For this review, take the finished solid that the model builds, in its own axes (mm). A direction names the side the tool comes from. Give positions to 0.01 mm unless a question says otherwise; leave off trailing zeros. Write each loop counter-clockwise with the first axis right and the second up, starting at its lowest first coordinate (ties: lowest second). Pieces come first, ordered by that corner, then holes.
Q1. Mouldability with a two-part tool opening along X and no side actions: class faces 4 (the conical face through (842.046, 6028.379, 11.443)), 5 (the flat face through (832, 5940.625, 5)), 6 (the flat face through (838.696, 5949.759, 11.61)) as released by +X, released by -X, zero draft, split by the parting line, or undercut.
Q2. We need section C-C (y = 6126.5). Write out the cut boundary in (x, z) (1 decimal), then the cut area to 3 significant figures.
Q3. We need section B-B (x = 865). Write out the cut boundary in (y, z) (3 decimals), then the cut area to 3 significant figures.
Q4. We need section A-A (y = 6048). Write out the cut boundary in (x, z), then the cut area to 3 significant figures.
Q5. For line 1 (Y direction, x = 835.5, z = 5); line 2 (Z direction, x = 841, y = 6138); line 3 (Y direction, x = 852, z = 4), list the stretches that pass through material, from the lowest coordinate up.
Q6. Machinability: for faces 1 (the cylindrical face through (839.37, 6142.44, 6.62)), 2 (the flat face through (864, 6173, 3.175)), 3 (the cylindrical face through (840.82, 6030.12, 4.79)), which of the approach directions +Z, -Z, +X, -X, +Y, -Y give a long, thin tool a straight path to every point of the face, cutting with its end or side? Answer none if there is none.
Q7. Insertion check: P1, Ø1, axis at y = 6009.5, z = 12, coming from the +X side; P2, Ø7, axis at x = 866, y = 6171.5, coming from the +Z side (3 decimals); P3, Ø4.5, axis at x = 830, z = 4.5, coming from the +Y side; P4, Ø5, axis at y = 6017, z = 11, coming from the -X side. Each pin has a flat end and moves straight along its axis. Give the tip position at first contact, or say it passes through.
```python
from build123d import *

# Parameters (mm, degrees)
SKETCH2_W                  = 82.738044028
SKETCH2_H                  = 243.598411898
BOSS_EXTRUDE1_DEPTH        = 3.175
BOSS_EXTRUDE2_DEPTH        = 243.598412
CUT_EXTRUDE1_DEPTH         = 6253.234293578
CUT_EXTRUDE1_DEPTH_BACK    = 6253.234293578
SKETCH3_W                  = 10.058364279
SKETCH3_H                  = 111.125
FILLET1_R                  = 6.35
CUT_EXTRUDE2_DEPTH         = 6243.564603497
DELETEFACE2_START          = 830.447299741
DELETEFACE2_OUTLINE_W      = 243.598411898
DELETEFACE2_OUTLINE_H      = 6
DELETEFACE2_DEPTH          = 0.551332964
F_6_0_204_DIAMETER_HOLE1_D = 5.1816
CUT_EXTRUDE3_START         = 3.175
CUT_EXTRUDE3_DEPTH         = 6231.095925463
SKETCH10_W                 = 38.1
SKETCH10_H                 = 3.175
BOSS_EXTRUDE4_DEPTH        = 6.35
BOSS_EXTRUDE6_DEPTH        = 1.5875
CUT_EXTRUDE4_DEPTH         = 913.829845298
FILLET2_R                  = 9.525
FILLET3_R                  = 3.175
SKETCH13_W                 = 8.255
SKETCH13_H                 = 6.35
BOSS_EXTRUDE5_DEPTH        = 1.5875
FILLET4_R                  = 2.54
FILLET5_SIZE               = 6.35
FILLET5_SIZE_2             = 3.175
FILLET6_R                  = 3.175
HOLE1_AT_2_COUNT           = 2
HOLE1_AT_2_PITCH           = 123.825
HOLE1_AT_3_COUNT           = 2
HOLE1_AT_3_PITCH           = 212.6865263
F_4_CLEARANCE_HOLE1_D      = 3.4544


# Read off the part's stored shape, not the designer's step: DeleteFace2
with BuildPart() as part:
    # Sketch2 → Boss-Extrude1 (new body)
    with BuildSketch(Plane.XY):
        with Locations((870.137648104, 6053.851709568)):
            Rectangle(SKETCH2_W, SKETCH2_H)
    extrude(amount=BOSS_EXTRUDE1_DEPTH)

    # Sketch5 → Boss-Extrude2 (add, through all)
    with BuildSketch(Plane(origin=(0, 6175.650915517, 0), x_dir=(1, 0, 0), z_dir=(0, 1, 0))):
        Polygon((828.76862609, -3.175), (840.781978058, -13.382293294), (845.472124982, -12.555293847), (843.81812609, -3.175), align=None)
    extrude(amount=-BOSS_EXTRUDE2_DEPTH)

    # Sketch3 → Cut-Extrude1 (cut, two sides: drawn at the far end of the back side and taken through both)
    with BuildSketch(Plane(origin=(1789.89403363, 0, -153.971769821), x_dir=(-0.9848077530122082, 0, 0.17364817766692958), z_dir=(-0.17364817766692958, 0, -0.9848077530122082)).offset(-CUT_EXTRUDE1_DEPTH_BACK)):
        with Locations((968.782821029, 6016.190003619)):
            Rectangle(SKETCH3_W, SKETCH3_H)
    extrude(amount=CUT_EXTRUDE1_DEPTH + CUT_EXTRUDE1_DEPTH_BACK, mode=Mode.SUBTRACT)

    # Fillet1
    fillet1_edges = [part.edges().sort_by_distance(p)[0] for p in [
        (839.602148372, 6071.752503619, 6.691146647),
        (839.602148372, 5960.627503619, 6.691146647),
    ]]
    fillet(fillet1_edges, radius=FILLET1_R)

    # Sketch4 → Cut-Extrude2 (cut, through all)
    with BuildSketch(Plane.XY.offset(3.175)):
        Polygon((843.81812609, 6170.570915517), (843.81812609, 6175.650915517), (911.506670118, 6175.650915517), (911.506670118, 5932.052503619), (905.156670118, 5932.052503619), (843.81812609, 5932.052503619), align=None)
    extrude(amount=-CUT_EXTRUDE2_DEPTH, mode=Mode.SUBTRACT)

    # DeleteFace2 outline → DeleteFace2 (cut)
    with BuildSketch(Plane(origin=(0, 0, 0), x_dir=(0, 1, 0), z_dir=(0.984807753012209, 0, -0.173648177666925)).offset(DELETEFACE2_START)):
        with Locations((6053.851709568, 148)):
            Rectangle(DELETEFACE2_OUTLINE_W, DELETEFACE2_OUTLINE_H)
    extrude(amount=DELETEFACE2_DEPTH, mode=Mode.SUBTRACT)

    # #6 (0.204) Diameter Hole1 (through all)
    with Locations(Plane(origin=(0, 0, 0), x_dir=(-1, 0, 0), z_dir=(0, 0, -1))):
        with Locations((-833.65812609, 6161.363415517), (-833.65812609, 6142.313415517), (-833.65812609, 5946.340003619)):
            Hole(F_6_0_204_DIAMETER_HOLE1_D / 2)

    # Sketch8 → Cut-Extrude3 (cut, through all)
    with BuildSketch(Plane.XY.offset(CUT_EXTRUDE3_START)):
        with BuildLine():
            Line((833.65812609, 6155.648415517), (828.76862609, 6155.648415517))
            ThreePointArc((828.76862609, 6155.648415517), (823.05362609, 6161.363415517), (828.76862609, 6167.078415517))
            Line((828.76862609, 6167.078415517), (833.65812609, 6167.078415517))
            ThreePointArc((833.65812609, 6167.078415517), (839.37312609, 6161.363415517), (833.65812609, 6155.648415517))
        make_face()
        with BuildLine():
            Line((833.65812609, 6136.598415517), (828.76862609, 6136.598415517))
            ThreePointArc((828.76862609, 6136.598415517), (823.05362609, 6142.313415517), (828.76862609, 6148.028415517))
            Line((828.76862609, 6148.028415517), (833.65812609, 6148.028415517))
            ThreePointArc((833.65812609, 6148.028415517), (839.37312609, 6142.313415517), (833.65812609, 6136.598415517))
        make_face()
        with BuildLine():
            Line((833.65812609, 5940.625003619), (828.76862609, 5940.625003619))
            ThreePointArc((828.76862609, 5940.625003619), (823.05362609, 5946.340003619), (828.76862609, 5952.055003619))
            Line((828.76862609, 5952.055003619), (833.65812609, 5952.055003619))
            ThreePointArc((833.65812609, 5952.055003619), (839.37312609, 5946.340003619), (833.65812609, 5940.625003619))
        make_face()
    extrude(amount=CUT_EXTRUDE3_DEPTH, mode=Mode.SUBTRACT)

    # Sketch10 → Boss-Extrude4 (add)
    with BuildSketch(Plane(origin=(0, 6175.650915517, 0), x_dir=(1, 0, 0), z_dir=(0, 1, 0))):
        with Locations((862.308287926, -1.5875)):
            Rectangle(SKETCH10_W, SKETCH10_H)
    extrude(amount=-BOSS_EXTRUDE4_DEPTH)

    # Sketch14 → Boss-Extrude6 (add)
    with BuildSketch(Plane(origin=(817.830939253, 0, -144.205660248), x_dir=(-0.17364817766692534, 0, -0.9848077530122089), z_dir=(0.9848077530122089, 0, -0.17364817766692534))):
        Polygon((-149.654244494, 6169.300915517), (-149.654244494, 6175.650915517), (-159.179244494, 6175.650915517), (-159.179244494, 5932.052503619), (-146.430265001, 5932.052503619), (-146.430265001, 6169.300915517), align=None)
    extrude(amount=BOSS_EXTRUDE6_DEPTH)

    # Sketch15 → Cut-Extrude4 (cut, through all)
    with BuildSketch(Plane(origin=(0, 6169.300915517, 0), x_dir=(1, 0, 0), z_dir=(0, 1, 0))):
        Polygon((843.258287926, 0), (844.870277672, 0), (844.821670234, 0.275666482), align=None)
    extrude(amount=-CUT_EXTRUDE4_DEPTH, mode=Mode.SUBTRACT)

    # Fillet2
    # the kernel refuses this fillet: 9.525 mm, written as the material it adds along each edge
    with BuildSketch(Plane(origin=(845.430115836, 6175.650915517, 3.175), x_dir=(1, 0, 0), z_dir=(0, -1, 0))) as fillet2_piece_1:
        with BuildLine():
            CenterArc((11.121110651, 9.525), FILLET2_R, 182.529491184, 87.470508816)
            Line((1.605391454, 9.104627365), (1.41507707, 9.096219913))
            ThreePointArc((1.41507707, 9.096219913), (0.61508985, 4.585393661), (-0.187605877, 0.033079978))
            Line((-0.187605877, 0.033079978), (0, -0.1905))
            Line((0, -0.1905), (11.121110651, -0.1905))
            Line((11.121110651, -0.1905), (11.121110651, 0))
        make_face()
    extrude(amount=6.35)

    # Fillet3
    # the kernel refuses this fillet: 3.175 mm, written as the material it adds along each edge
    with BuildSketch(Plane(origin=(847.03550729, 6169.300915517, 12.279627365), x_dir=(0.9848077530122001, 0, -0.17364817766697505), z_dir=(-0.17364817766697507, 0, -0.9848077530122002))) as fillet3_piece_1_section:
        with BuildLine():
            CenterArc((FILLET3_R, FILLET3_R), FILLET3_R, 180, 90)
            Line((0, FILLET3_R), (0, 0))
            Line((0, 0), (FILLET3_R, 0))
        make_face()
    fillet3_piece_1 = extrude(amount=20.406560411, mode=Mode.PRIVATE)
    fillet3_piece_1 = fillet3_piece_1 - Plane(origin=(856.551226487, 6168.523076842, 12.7), x_dir=(1, 0, 0), z_dir=(0, 1, 0)) * Cylinder(9.525, 54, mode=Mode.PRIVATE)
    fillet3_piece_1 = split(fillet3_piece_1, bisect_by=Plane(origin=(846.439228991, 6168.523076842, 0), z_dir=(0, 0, 1)), keep=Keep.TOP, mode=Mode.PRIVATE)
    add(fillet3_piece_1)

    # Sketch13 → Boss-Extrude5 (add)
    with BuildSketch(Plane.XY.offset(3.175)):
        with Locations((877.230787926, 6172.475915517)):
            Rectangle(SKETCH13_W, SKETCH13_H)
    extrude(amount=BOSS_EXTRUDE5_DEPTH)

    # Fillet4
    # the kernel refuses this fillet: 2.54 mm, written as the material it adds along each edge
    with BuildSketch(Plane(origin=(873.103287926, 6175.650915517, 3.175), x_dir=(-1, 0, 0), z_dir=(0, -1, 0))) as fillet4_piece_1:
        with BuildLine():
            CenterArc((2.35464302, -2.54), FILLET4_R, 90, 67.975687163)
            Line((0, -1.5875), (-0.04709286, -1.56845))
            ThreePointArc((-0.04709286, -1.56845), (-0.0508, -0.79375), (-0.0508, 0))
            Line((-0.0508, 0), (0, 0.0508))
            Line((0, 0.0508), (2.35464302, 0.0508))
            Line((2.35464302, 0.0508), (2.35464302, 0))
        make_face()
    extrude(amount=6.35)

    # Fillet5
    # an asymmetric fillet: 6.35, 3.175 mm, written as the material it takes off along each edge
    with BuildSketch(Plane(origin=(849.79217211, 5932.052503619, 27.913450444), x_dir=(-0.9848077530122089, 0, 0.17364817766692534), z_dir=(-0.17364817766692536, 0, -0.984807753012209))) as fillet5_piece_1:
        with BuildLine():
            Bezier((FILLET5_SIZE, 0), (0, 0), (0, FILLET5_SIZE_2), weights=[1, 0.707106781, 1])
            Line((0, FILLET5_SIZE_2), (0, 0))
            Line((0, 0), (FILLET5_SIZE, 0))
        make_face()
    extrude(amount=44.219060411, mode=Mode.SUBTRACT)

    # Fillet6
    # the kernel refuses this fillet: 3.175 mm, written as the material it takes off along each edge
    with BuildSketch(Plane(origin=(828.76862609, 6175.650915517, -7.9375), x_dir=(1, 0, 0), z_dir=(0, 0, 1))) as fillet6_piece_1:
        with BuildLine():
            CenterArc((FILLET6_R, -FILLET6_R), FILLET6_R, 90, 90)
            Line((0, -FILLET6_R), (0, 0))
            Line((0, 0), (FILLET6_R, 0))
        make_face()
    extrude(amount=19.05, mode=Mode.SUBTRACT)
    with BuildSketch(Plane(origin=(828.76862609, 5932.052503619, -7.9375), x_dir=(1, 0, 0), z_dir=(0, 0, 1)), Plane(origin=(828.76862609, 5960.627503619, -7.9375), x_dir=(0, -1, 0), z_dir=(0, 0, 1)), Plane(origin=(828.76862609, 6071.752503619, 11.1125), x_dir=(0, 1, 0), z_dir=(0, 0, -1))) as fillet6_piece_2:
        with BuildLine():
            CenterArc((FILLET6_R, FILLET6_R), FILLET6_R, 180, 90)
            Line((0, FILLET6_R), (0, 0))
            Line((0, 0), (FILLET6_R, 0))
        make_face()
    extrude(amount=19.05, mode=Mode.SUBTRACT)
    with BuildSketch(Plane(origin=(881.358287926, 6175.650915517, -7.9375), x_dir=(-1, 0, 0), z_dir=(0, 0, 1))) as fillet6_piece_3:
        with BuildLine():
            CenterArc((FILLET6_R, FILLET6_R), FILLET6_R, 180, 90)
            Line((0, FILLET6_R), (0, 0))
            Line((0, 0), (FILLET6_R, 0))
        make_face()
    extrude(amount=20.6375, mode=Mode.SUBTRACT)

    # Sketch17 → Hole1 (revolve, cut)
    with BuildSketch(Plane(origin=(843.908742674, 6153.425915517, 12.830960329), x_dir=(0.9848077530122085, 0, -0.17364817766692853), z_dir=(0, 1, 0))):
        Polygon((0, 0), (0, 3.429), (1.9431, 3.429), (2.0701, 0), align=None)
    hole1 = revolve(axis=Axis((824.807443131, 6153.425915517, -95.497892502), (0.1736481776669289, 0, 0.9848077530122084)), mode=Mode.SUBTRACT)

    # Hole1 at 2: Hole1 ×2
    with Locations(*[(0, -i * HOLE1_AT_2_PITCH, 0) for i in range(1, HOLE1_AT_2_COUNT)]):
        add(hole1, mode=Mode.SUBTRACT)

    # Hole1 at 3: Hole1 ×2
    with Locations(*[(0, -i * HOLE1_AT_3_PITCH, 0) for i in range(1, HOLE1_AT_3_COUNT)]):
        add(hole1, mode=Mode.SUBTRACT)

    # #4 Clearance Hole1 (through all)
    with Locations(Plane(origin=(27.641185729, 0, 156.760954096), x_dir=(0.9848077530122085, 0, -0.17364817766692853), z_dir=(0.17364817766692853, 0, 0.9848077530122085))):
        with Locations((828.859799741, 5940.739389217), (828.859799741, 6029.600915517), (828.859799741, 6153.425915517)):
            Hole(F_4_CLEARANCE_HOLE1_D / 2)


solid = part.part
```
Computed:
1. face 4: undercut
1. face 5: zero draft
1. face 6: released by -X
2. outline: (828.8, 0) - (844.9, 0) - (847, 12.3) - (840.8, 13.4) - (828.8, 3.2) - close
2. area: 166 mm2
3. outline: (6169.301, 0) - (6175.651, 0) - (6175.651, 3.175) - (6169.301, 3.175) - close
3. area: 20.2 mm2
4. outline: (838.42, 0) - (844.87, 0) - (847.04, 12.28) - (840.78, 13.38) - close
4. area: 82.7 mm2
5. line 1: y = 5932.05 to 5940.93, 5951.75 to 5961.19, 6071.19 to 6136.9, 6147.72 to 6155.95, 6166.77 to 6175.65
5. line 2: z = 0 to 13.34
5. line 3: y = 6169.3 to 6175.65
6. face 1: +Z, -X
6. face 2: +Z, +Y, -Y
6. face 3: none
7. P1: stops at x = 847.04
7. P2: stops at z = 3.175
7. P3: stops at y = 6175.65
7. P4: stops at x = 839.92
